Answer from the drawing. Dimensions are ordinates in mm from the lowest x, y and z of the part. Coordinates: 2 decimals unless noted, no trailing zeros. Write each loop counter-clockwise with the first axis right and the second up, starting at its lowest first coordinate (ties: lowest second). Pieces come first, ordered by that corner, then holes. Notation, with made-up numbers: (-26, 71) -> (-5, 71) arc R15 ccw to (-5, 88) -> close; hole circle Ø10 at (-2, 35). An arc over 180 degrees is marked (long way). One line per item, written item: value. Start each with the question number.
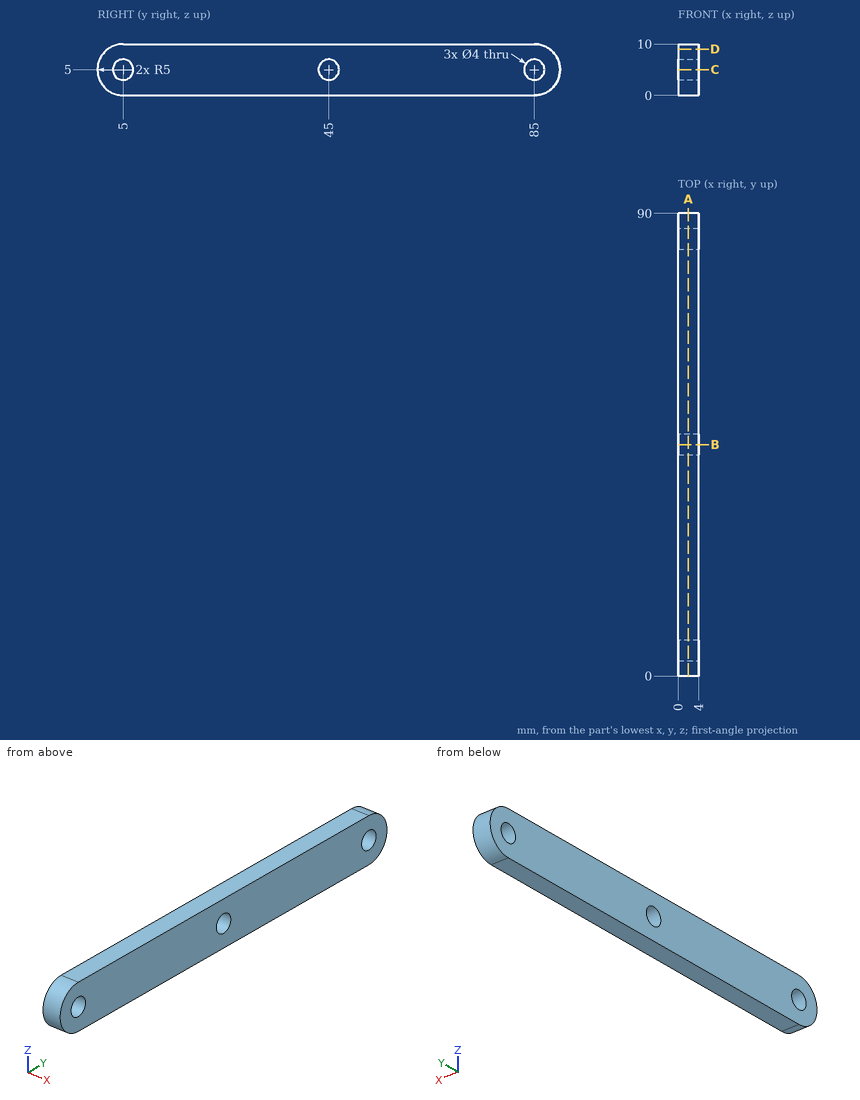
1. A cutting plane is placed at B-B on y = 45. Give the vertices of the cut face in (x, z).
2. A cutting plane is placed at D-D on z = 9. Give the vertices of the cut face in (x, y).
3. A cutting plane is placed at C-C on z = 5. Give the vertices of the cut face in (x, y), then the cut area to 3 significant figures.
4. Find the intervals of material crossed by probe 1 along Y at (x, z) = (2, 4.75); probe 2 along Y at (x, z) = (1.3, 3.75); probe 3 along Z at (x, y) = (3, 5), in increasing order. Write a range as from..to.
5. Given pin 1 (3 mm diameter, centred on y = 45, z = 5, fed in from -X); pin 2 (1 mm diameter, centred on x = 1, z = 6, fed in from +Y); pin 3 (1 mm diameter, centred on x = 1, z = 9, fed in from -Y), each flat-ended and moving along its own axis, determine where each tip first touches the part or whether it passes through.
6. A cutting plane is placed at A-A on x = 2. Give the vertices of the cut face in (y, z), then the cut area to 3 significant figures.
Derived:
1. outline: (0, 0) -> (4, 0) -> (4, 3) -> (0, 3) -> close; (0, 7) -> (4, 7) -> (4, 10) -> (0, 10) -> close
2. outline: (0, 2) -> (4, 2) -> (4, 88) -> (0, 88) -> close
3. outline: (0, 0) -> (4, 0) -> (4, 3) -> (0, 3) -> close; (0, 7) -> (4, 7) -> (4, 43) -> (0, 43) -> close; (0, 47) -> (4, 47) -> (4, 83) -> (0, 83) -> close; (0, 87) -> (4, 87) -> (4, 90) -> (0, 90) -> close
3. area: 312 mm2
4. probe 1: y = 0.01..3.02, 6.98..43.02, 46.98..83.02, 86.98..89.99
4. probe 2: y = 0.16..3.44, 6.56..43.44, 46.56..83.44, 86.56..89.84
4. probe 3: z = 0..3, 7..10
5. pin 1: passes through
5. pin 2: stops at y = 89.97
5. pin 3: stops at y = 1.43
6. outline: (5, 0) -> (85, 0) arc R5 ccw to (85, 10) -> (5, 10) arc R5 ccw to start; hole circle Ø4 at (5, 5); hole circle Ø4 at (45, 5); hole circle Ø4 at (85, 5)
6. area: 841 mm2
